Can you work these out from the model? Positions are in its coordinate system, mm. A direction names the side the tool comes from. Round coordinates to 2 decimals unless told otherwise and drop trailing zeros. Loops run counter-clockwise (first coordinate to the right, second up) from the corner with the lowest first, then second, coordinate; pieces in that order, holes last. Notation, with made-up numbers: (74.5, 12) -> (79.5, 12) arc R31 ccw to (79.5, 37) -> close; hole circle Ø4 at (6.5, -23.5). An arc over 180 degrees is marked (long way). Use a Markdown table: item, result.
Autodesk Inventor part; units mm, degrees
ref_plane "YZ Plane" through (0, 0, 0) normal (1, 0, 0) x (0, 1, 0)
ref_plane "XZ Plane" through (0, 0, 0) normal (0, 1, 0) x (-1, 0, 0)
ref_plane "XY Plane" through (0, 0, 0) normal (0, 0, 1) x (1, 0, 0)
sketch "Sketch1" plane through (0, 0, 0) normal (0, 0, 1) x (1, 0, 0)
  circle A0 centre (0, 0) radius 10
  circle A1 centre (0, 0) radius 20
  line L0 (-15, 0) -> (15, 0)
  line L1 (15, 0) -> (15, 50)
  line L2 (15, 50) -> (-15, 50)
  line L3 (-15, 50) -> (-15, 0)
  point P0 (-15, 13.2288)
  point P1 (15, 13.2288)
  dimension "d0" = 20
  dimension "d1" = 40
  dimension "d2" = 30
  dimension "d3" = 50
extrude "Extrusion1" add sketch "Sketch1" along normal blind 20
sketch "Sketch2" plane through (0, 0, 20) normal (0, 0, 1) x (1, 0, 0)
  circle A0 centre (0, 0) radius 10
  dimension "d6" = 20
extrude "Extrusion2" cut sketch "Sketch2" against normal blind 15
sketch "Sketch4" plane through (-15, 13.2288, 0) normal (-1, 0, 0) x (0, 0, 1)
  line L0 (0, 36.7712) -> (20, 36.7712)
  line L1 (0, 0) -> (0, 36.7712)
  line L2 (20, 36.7712) -> (0, 36.7712)
  line L3 (0, 36.7712) -> (0, 0)
  line L4 (0, 0) -> (20, 0)
  line L5 (20, 0) -> (20, 36.7712)
  line L6 (0, 0) -> (20, 0)
  line L7 (20, 36.7712) -> (10, 36.7712)
  line L8 (10, 36.7712) -> (10, 0)
  line L9 (10, 0) -> (20, 0)
  line L10 (20, 0) -> (20, 36.7712)
  line L11 (10, 0) -> (16, 0)
  line L12 (16, 0) -> (16, 25)
  line L13 (16, 25) -> (10, 25)
  line L14 (10, 25) -> (10, 0)
  line L15 (10, 25) -> (4, 25)
  line L16 (4, 25) -> (4, 0)
  line L17 (4, 0) -> (10, 0)
  line L18 (10, 0) -> (10, 25)
  line L19 (4, 25) -> (16, 25)
  line L20 (16, 25) -> (16, 30.0005)
  line L21 (16, 30.0005) -> (4, 30.0005)
  line L22 (4, 30.0005) -> (4, 25)
  line L23 (4, 30.0005) -> (16, 30.0005)
  line L24 (16, 30.0005) -> (16, 7.0005)
  line L25 (16, 7.0005) -> (4, 7.0005)
  line L26 (4, 7.0005) -> (4, 30.0005)
  line L27 (10, 7.0005) -> (16, 7.0005)
  line L28 (16, 7.0005) -> (16, 0)
  line L29 (16, 0) -> (10, 0)
  line L30 (10, 0) -> (10, 7.0005)
  point P0 (0, -13.2288)
  dimension "d13" = 6
  dimension "d14" = 25
  dimension "d15" = 6
  dimension "d16" = 23
extrude "Extrusion3" cut sketch "Sketch4" against normal blind 23 contours L21 L20 L13 L8 | L8 L15 L22 L21 | L13 L12 L25 L8 | L8 L25 L16 L15
sketch "Sketch6" plane through (-15, 13.2288, 0) normal (-1, 0, 0) x (0, 0, 1)
  line L0 (4, 7.0005) -> (4, 30.0005)
  line L1 (4, 7.0005) -> (16, 7.0005)
  line L2 (16, 7.0005) -> (16, 2.2005)
  line L3 (16, 2.2005) -> (4, 2.2005)
  line L4 (4, 2.2005) -> (4, 7.0005)
  line L5 (4, 30.0005) -> (16, 30.0005)
  line L6 (16, 30.0005) -> (16, 34.8005)
  line L7 (16, 34.8005) -> (4, 34.8005)
  line L8 (4, 34.8005) -> (4, 30.0005)
  point P0 (0, -13.2288)
  dimension "d19" = 12
  dimension "d20" = 4.8
  dimension "d21" = 4.8
extrude "Extrusion4" cut sketch "Sketch6" against normal blind 16
sketch "Sketch7" plane through (1, 13.2288, 0) normal (-1, 0, 0) x (0, 0, 1)
  line L0 (4, 30.0005) -> (16, 30.0005)
  line L1 (4, 30.0005) -> (10, 30.0005)
  line L2 (10, 30.0005) -> (10, 32.5005)
  line L3 (10, 32.5005) -> (4, 32.5005)
  line L4 (4, 32.5005) -> (4, 30.0005)
  circle A0 centre (10, 32.5005) radius 0.75
  line L5 (16, 7.0005) -> (4, 7.0005)
  line L6 (16, 7.0005) -> (16, 2.2005)
  line L7 (4, 7.0005) -> (16, 7.0005)
  line L8 (16, 7.0005) -> (16, 4.5005)
  line L9 (16, 4.5005) -> (4, 4.5005)
  line L10 (4, 4.5005) -> (4, 7.0005)
  line L11 (10, 4.5005) -> (4, 4.5005)
  line L12 (4, 4.5005) -> (4, 7.0005)
  line L13 (4, 7.0005) -> (10, 7.0005)
  line L14 (10, 7.0005) -> (10, 4.5005)
  circle A1 centre (10, 4.5005) radius 0.75
  point P0 (0, -13.2288)
  dimension "d24" = 2.5
  dimension "d25" = 1.5
  dimension "d26" = 2.5
  dimension "d27" = 1.5
extrude "Extrusion5" cut sketch "Sketch7" against normal blind 8 contours A0 L3 L2 | L2 L3 A0 | A1 L9 L14 | L14 L9 A1 | A1 L9
sketch "Sketch8" plane through (15, 13.2288, 0) normal (1, 0, 0) x (0, 0, -1)
  line L0 (0, 36.7712) -> (0, 0)
  line L1 (-20, 36.7712) -> (-20, 0)
  line L2 (0, 36.7712) -> (-20, 36.7712)
  line L3 (-20, 36.7712) -> (-20, 26.7712)
  line L4 (-20, 26.7712) -> (0, 26.7712)
  line L5 (0, 26.7712) -> (0, 36.7712)
  line L6 (0, 26.7712) -> (-20, 26.7712)
  line L7 (-20, 26.7712) -> (-20, 18.7712)
  line L8 (-20, 18.7712) -> (0, 18.7712)
  line L9 (0, 18.7712) -> (0, 26.7712)
  line L10 (0, 26.7712) -> (-10, 26.7712)
  line L11 (-10, 26.7712) -> (-10, 18.7712)
  line L12 (-10, 18.7712) -> (0, 18.7712)
  line L13 (0, 18.7712) -> (0, 26.7712)
  line L14 (-10, 26.7712) -> (-5, 26.7712)
  line L15 (-5, 26.7712) -> (-5, 22.7712)
  line L16 (-5, 22.7712) -> (-10, 22.7712)
  line L17 (-10, 22.7712) -> (-10, 26.7712)
  line L18 (-10, 22.7712) -> (-15, 22.7712)
  line L19 (-15, 22.7712) -> (-15, 26.7712)
  line L20 (-15, 26.7712) -> (-10, 26.7712)
  line L21 (-10, 26.7712) -> (-10, 22.7712)
  point P0 (0, -13.2288)
  dimension "d30" = 10
  dimension "d31" = 8
  dimension "d32" = 5
  dimension "d33" = 5
extrude "Extrusion6" cut sketch "Sketch8" against normal blind 15.8125 contours L15 L16 L11 L4 | L11 L18 L19 L4
sketch "Sketch9" plane through (0, 0, 5) normal (0, 0, 1) x (1, 0, 0)
  circle A0 centre (0, 0) radius 1
  circle A1 centre (7, 0) radius 1.5
  circle A2 centre (0, 0) radius 1.5
  circle A3 centre (-7, 0) radius 1.5
  dimension "d36" = 2
  dimension "d37" = 3
  dimension "d38" = 3
  dimension "d39" = 3
extrude "Extrusion7" cut sketch "Sketch9" against normal blind 8 contours A0 | A1 | A2 | A3
sketch "Sketch10" plane through (-15, 50, 0) normal (0, 1, 0) x (1, 0, 0)
  line L0 (0, 0) -> (0, -20)
  line L1 (0, 0) -> (29.4792, 0)
  line L2 (29.4792, 0) -> (29.4792, -20)
  line L3 (29.4792, -20) -> (0, -20)
  line L4 (0, -20) -> (0, 0)
  point P0 (15, 0)
extrude "Extrusion8" add sketch "Sketch10" along normal blind 10
sketch "Sketch11" plane through (0, 0, 0) normal (0, 0, -1) x (-1, 0, 0)
  line L0 (15, 13.2288) -> (15, 60)
  line L1 (-15, 13.2288) -> (-15, 50)
  line L2 (15, 60) -> (-15, 60)
  line L3 (-15, 60) -> (-15, 45)
  line L4 (-15, 45) -> (15, 45)
  line L5 (15, 45) -> (15, 60)
  line L6 (15, 45) -> (-15, 45)
  line L7 (-15, 45) -> (-15, 35)
  line L8 (-15, 35) -> (15, 35)
  line L9 (15, 35) -> (15, 45)
  point P0 (0, 0)
  dimension "d47" = 15
  dimension "d48" = 10
sketch "Sketch12" plane through (14.4792, 50, 20) normal (1, 0, 0) x (0, 0, -1)
  line L0 (20, 0) -> (20, 10)
  line L1 (0, 0) -> (20, 0)
  line L2 (20, 0) -> (20, 10)
  line L3 (20, 10) -> (0, 10)
  line L4 (0, 10) -> (0, 0)
  point P0 (20, -50)
extrude "Extrusion9" cut sketch "Sketch12" against normal blind 59.6125
sketch "Sketch13" plane through (-15, 50, 0) normal (0, 1, 0) x (1, 0, 0)
  line L0 (30, 0) -> (30, -20)
  line L1 (0, 0) -> (30, 0)
  line L2 (30, 0) -> (30, -20)
  line L3 (30, -20) -> (0, -20)
  line L4 (0, -20) -> (0, 0)
  point P0 (15, 0)
extrude "Extrusion10" add sketch "Sketch13" along normal blind 10
extrude "Extrusion11" add sketch "Sketch11" along normal blind 10
sketch "Sketch15" plane through (0, 0, 20) normal (0, 0, 1) x (1, 0, 0)
  line L0 (-15, 60) -> (15, 60)
  line L1 (-15, 60) -> (0, 60)
  line L2 (0, 60) -> (0, 35)
  line L3 (0, 35) -> (-15, 35)
  line L4 (-15, 35) -> (-15, 60)
  point P0 (0, 0)
  dimension "d56" = 25
extrude "Extrusion12" add sketch "Sketch15" along normal blind 10
sketch "Sketch16" plane through (0, 0, -10) normal (0, 0, -1) x (-1, 0, 0)
  line L0 (-15, 13.2288) -> (-15, 60)
  line L1 (0, 35) -> (15, 35)
  line L2 (-15, 60) -> (0, 60)
  line L3 (0, 60) -> (0, 35)
  line L4 (0, 35) -> (-15, 35)
  line L5 (-15, 35) -> (-15, 60)
  point P0 (0, 0)
extrude "Extrusion13" cut sketch "Sketch16" against normal blind 10
sketch "Sketch18" plane through (0, 0, 20) normal (0, 0, 1) x (1, 0, 0)
  circle A0 centre (0, 0) radius 10
extrude "Extrusion15" add sketch "Sketch18" against normal blind 16
sketch "Sketch19" plane through (0, 0, 0) normal (0, 0, -1) x (-1, 0, 0)
  circle A0 centre (0, 0) radius 1.5
  circle A1 centre (0, 0) radius 10
  dimension "d72" = 20
extrude "Extrusion16" cut sketch "Sketch19" against normal blind 16
sketch "Sketch20" plane through (0, 0, 4) normal (0, 0, -1) x (-1, 0, 0)
  circle A0 centre (0, 0) radius 1.5
  circle A1 centre (0, 0) radius 1.5
extrude "Extrusion17" cut sketch "Sketch20" against normal blind 30.0375
sketch "Sketch21" plane through (0, 0, 16) normal (0, 0, -1) x (-1, 0, 0)
  circle A0 centre (5, 0) radius 1
  circle A1 centre (-5, 0) radius 1
  point P0 (0, 0)
  dimension "d77" = 2
  dimension "d78" = 2
extrude "Extrusion18" cut sketch "Sketch21" against normal blind 138.2375
chamfer "Chamfer2" distance 8 angle 45 1 edges at (10, 0, 0)
sketch "Sketch22" plane through (-15, 13.2288, 0) normal (-1, 0, 0) x (0, 0, 1)
  circle A0 centre (-4, 36.7712) radius 2
  circle A1 centre (-4, 36.7712) radius 2
  circle A2 centre (24, 36.7712) radius 2
  circle A3 centre (24, 36.7712) radius 2
  point P0 (0, -13.2288)
sketch "Sketch25" plane through (-15, 13.2288, 0) normal (-1, 0, 0) x (0, 0, 1)
  circle A0 centre (-4, 36.7712) radius 2
  circle A1 centre (-4, 36.7712) radius 8
  arc A2 (7.7087, 23.1005) -> (12.2913, 23.1005) centre (10, 24.1005) ccw
  circle A3 centre (10, 24.1005) radius 8
  circle A4 centre (24, 36.7712) radius 2
  circle A5 centre (24, 36.7712) radius 8
  circle A6 centre (-4, 36.7712) radius 2
  circle A7 centre (24, 36.7712) radius 2
  line L0 (-4, 36.7712) -> (24.7591, 36.7712)
  line L1 (24.7591, 36.7712) -> (24.7591, 61.7712)
  line L2 (24.7591, 61.7712) -> (-4, 61.7712)
  line L3 (-4, 61.7712) -> (-4, 36.7712)
  point P0 (0, -13.2288)
  dimension "d92" = 16
  dimension "d93" = 16
  dimension "d94" = 16
  dimension "d99" = 25
sketch "Sketch29" plane through (-15, 15.4292, 4) normal (0, 0, 1) x (1, 0, 0)
  point P0 (15, -15.4292)
sketch "Sketch33" plane through (15, 13.2288, 20) normal (1, 0, 0) x (0, 0, -1)
  line L0 (5, 26.7712) -> (5, 22.7712)
  line L1 (5, 26.7712) -> (15, 26.7712)
  line L2 (15, 26.7712) -> (15, 34.7712)
  line L3 (15, 34.7712) -> (5, 34.7712)
  line L4 (5, 34.7712) -> (5, 26.7712)
  point P0 (20, -13.2288)
  dimension "d110" = 10
  dimension "d111" = 8
extrude "Extrusion27" cut sketch "Sketch33" against normal blind 7
sketch "Sketch34" plane through (0, 0, 30) normal (0, 0, 1) x (1, 0, 0)
  point P0 (0, 0)
sketch "Sketch37" plane through (0, 0, 30) normal (0, 0, 1) x (1, 0, 0)
  point P0 (0, 0)
sketch "Sketch38" plane through (-15, 13.2288, 0) normal (-1, 0, 0) x (0, 0, 1)
  point P0 (0, -13.2288)
sketch "Sketch41" plane through (-15, 13.2288, 0) normal (-1, 0, 0) x (0, 0, 1)
  line L0 (30, 21.7712) -> (30, 46.7712)
  line L1 (30, 21.7712) -> (20, 21.7712)
  line L2 (20, 21.7712) -> (20, 48.4389)
  line L3 (20, 48.4389) -> (30, 48.4389)
  line L4 (30, 48.4389) -> (30, 21.7712)
  point P0 (0, -13.2288)
extrude "Extrusion31" cut sketch "Sketch41" against normal blind 36.0375
sketch "Sketch42" plane through (0, 0, -10) normal (0, 0, -1) x (-1, 0, 0)
  line L0 (0, 35) -> (15, 35)
  line L1 (0, 60) -> (0, 35)
  line L2 (15, 35) -> (0, 35)
  line L3 (0, 35) -> (0, 60)
  line L4 (0, 60) -> (15, 60)
  line L5 (15, 60) -> (15, 35)
  point P0 (0, 0)
extrude "Extrusion32" add sketch "Sketch42" along normal blind 5
sketch "Sketch43" plane through (-15, 35, 0) normal (0, -1, 0) x (1, 0, 0)
  line L0 (15, -15) -> (15, 0)
  line L1 (0, 0) -> (15, 0)
  line L2 (15, -15) -> (0, -15)
  line L3 (0, -15) -> (0, 0)
  line L4 (0, 0) -> (15, 0)
  line L5 (15, 0) -> (15, -15)
extrude "Extrusion33" add sketch "Sketch43" along normal blind 10
sketch "Sketch44" plane through (-15, 13.2288, 0) normal (-1, 0, 0) x (0, 0, 1)
  line L0 (16, 2.2005) -> (4, 2.2005)
  line L1 (10, 2.2005) -> (10, 34.6918)
  circle A0 centre (10, 24.0854) radius 8
  line L2 (10, 24.0854) -> (-8, 24.0854)
  circle A1 centre (-8, 24.0854) radius 8
  circle A2 centre (-8, 24.0854) radius 2.5
  point P0 (0, -13.2288)
  dimension "d128" = 16
  dimension "d129" = 18
  dimension "d130" = 16
  dimension "d131" = 5
extrude "Extrusion34" add sketch "Sketch44" along normal blind 6 contours A2
sketch "Sketch45" plane through (-15, 60, 0) normal (0, 1, 0) x (1, 0, 0)
  line L0 (0, 0) -> (0, 15)
  line L1 (0, -20) -> (30, -20)
  line L2 (0, 15) -> (15, 15)
  line L3 (15, 15) -> (15, -20)
  line L4 (15, -20) -> (0, -20)
  line L5 (0, -20) -> (0, 15)
  line L6 (30, -20) -> (30, 0)
  line L7 (15, 0) -> (30, 0)
  line L8 (30, 0) -> (30, -20)
  line L9 (30, -20) -> (15, -20)
  line L10 (15, -20) -> (15, 0)
extrude "Extrusion35" cut sketch "Sketch45" against normal blind 7
properties part number "NeWConcept"
1. I want a section at C-C (y = 29). Please give me the cut outline in (x, z).
Answer sheet:
| item | result |
|---|---|
| outline | (-15, -15) -> (0, -15) -> (0, 0) -> (15, 0) -> (15, 20) -> (-15, 20) -> (-15, 16) -> (8, 16) -> (8, 4) -> (-15, 4) -> close |
2. Which directions (+Z, -Z, +X, -X, +Y, -Y) give clear straight access to the entire face, cutting with the end or side of a thin tool? Please do faces 4 (the flat face through (-2, 0, 16)), 5 (the flat face through (-8, 25, -7)), 6 (the flat face through (12, 36, 10)), 7 (the flat face through (-7, 48.029, 10)), 8 (the flat face through (12, 42, 15)).
Answer sheet:
| item | result |
|---|---|
| face 4 | -Z |
| face 5 | -Z, +X, -X, -Y |
| face 6 | +X, -X |
| face 7 | -X |
| face 8 | +X |
3. I want a section at D-D (z = 1.5). Please give me the cut outline in (x, y).
Answer sheet:
| item | result |
|---|---|
| outline | (-15, 13.23) arc R20 ccw (long way) to (15, 13.23) -> (15, 53) -> (-15, 53) -> close; hole circle Ø33 at (0, 0) |
4. I need wall thicknesses on line 1 (Y direction, x = 0, z = 12); line 2 (Z direction, x = -3, y = 18); line 3 (Z direction, x = -4, y = 33). Which ranges of each line are inside material? Lowest first, please.
Answer sheet:
| item | result |
|---|---|
| line 1 | y = -20 to -10, 10 to 15.43, 48.03 to 53 |
| line 2 | z = 0 to 4, 16 to 20 |
| line 3 | z = -15 to 4, 16 to 20 |
5. Will these pins go through, and if not, where does the flat tip stop? pin 1 Ø4 at (x, z) = (-5, -8.5) entering from -Y; pin 2 Ø2 at (y, z) = (26, -11.5) entering from -X; pin 3 Ø2 at (x, z) = (11.5, 8) entering from -Y.
Answer sheet:
| item | result |
|---|---|
| pin 1 | stops at y = 25 |
| pin 2 | stops at x = -15 |
| pin 3 | stops at y = -17.02 |
6. I want a section at A-A (z = 10). Please give me the cut outline in (x, y).
Answer sheet:
| item | result |
|---|---|
| outline | (-15, 13.23) arc R20 ccw (long way) to (15, 13.23) -> (15, 36) -> (8, 36) -> (8, 20.23) -> (1, 20.23) -> (1, 18.48) -> (9, 18.48) -> (9, 16.98) -> (1, 16.98) -> (1, 15.43) -> (-15, 15.43) -> close; (-15, 48.03) -> (1, 48.03) -> (1, 46.48) -> (8, 46.48) -> (8, 48) -> (15, 48) -> (15, 53) -> (-15, 53) -> close; (1, 43.23) -> (8, 43.23) -> (8, 44.98) -> (1, 44.98) -> close; hole circle Ø20 at (0, 0) |
7. I want a section at B-B (y = 0). Please give me the cut outline in (x, z).
Answer sheet:
| item | result |
|---|---|
| outline | (-20, 0) -> (-18, 0) -> (-10, 8) -> (-10, 16) -> (-6, 16) -> (-6, 20) -> (-20, 20) -> close; (-4, 16) -> (-1.5, 16) -> (-1.5, 20) -> (-4, 20) -> close; (1.5, 16) -> (4, 16) -> (4, 20) -> (1.5, 20) -> close; (6, 16) -> (10, 16) -> (10, 8) -> (18, 0) -> (20, 0) -> (20, 20) -> (6, 20) -> close |
8. If we mould it in two halves opening along Y, with no side actions, what happens to faces 1 (the flat face through (15, 33, 10)), 2 (the cylindrical face through (-17.958, 39.755, -8.542)), 3 (the flat face through (8, 47, 10))? For each: +Y half, -Y half, draft (parallel to the pull), parting line (faces both ways), or undercut.
Answer sheet:
| item | result |
|---|---|
| face 1 | draft |
| face 2 | parting line |
| face 3 | undercut |
